from build123d import *

# Parameters (mm, degrees)
F0_W     = 100
F0_H     = 50
F1_DEPTH = 5
F2_W     = 5
F2_H     = 5
F3_DEPTH = 5
F4_W     = 5
F4_H     = 5
F5_DEPTH = 5
F6_W     = 5
F6_H     = 5
F7_DEPTH = 5


with BuildPart() as f1:
    # F0 (on Top) → F1 (new body)
    with BuildSketch(Plane.XY):
        Rectangle(F0_W, F0_H)
    extrude(amount=F1_DEPTH)

    # F2 (on face) → F3 (join)
    with BuildSketch(Plane(origin=(0, 25, 0), x_dir=(-1, 0, 0), z_dir=(0, 1, 0))):
        with Locations((0, -2.5)):
            Rectangle(F2_W, F2_H)
    extrude(amount=-F3_DEPTH)

    # F4 (on face) → F5 (join)
    with BuildSketch(Plane.XZ.offset(25)):
        with Locations((0, -2.5)):
            Rectangle(F4_W, F4_H)
    extrude(amount=-F5_DEPTH)

    # F6 (on face) → F7 (cut, through all)
    with BuildSketch(Plane.XY.offset(5)):
        Polygon((-50, 2.5), (-50, 0), (-50, -2.5), (-45, -2.5), (-45, 2.5), align=None)
        with Locations((-32.5, 0)):
            Rectangle(F6_W, F6_H)
        with Locations((32.5, 0)):
            Rectangle(F6_W, F6_H)
        Polygon((45, 2.5), (45, -2.5), (50, -2.5), (50, 0), (50, 2.5), align=None)
    extrude(amount=-F7_DEPTH, mode=Mode.SUBTRACT)


solid = f1.part
Read the model definition and answer for the solid it produces. Units are mm, in the model's axes. A direction names the side the tool comes from. Coordinates: 2 decimals unless noted, no trailing zeros. Order: outer loops, then holes, each group sorted by start corner. A loop starts at its lowest first (then second) coordinate and runs counter-clockwise, first axis right, second up. Notation, with made-up numbers: (28.25, 36.25) -> (55.25, 36.25) arc R20 cw to (55.25, 64.25) -> close; hole circle Ø1 at (-25, 50). An arc over 180 degrees is marked (long way). Answer as a JSON object with one key per item and string values.
1) Consider line 1 along Y through (x, z) = (-34.5, 4.75); line 2 along Z through (x, y) = (25.5, 12.5); line 3 along X through (y, z) = (21.5, -3.5). Determine where each line is inside the solid, lowest interval first. Write a range as from..to.
Model answer:
{"line 1": "y = -25..-2.5, 2.5..25", "line 2": "z = 0..5", "line 3": "x = -2.5..2.5"}
2) A tool of negligible diameter and unlimited length cuts with its end or side. For faces 1 (the face through (2.5, -23, -3)), 2 (the face through (48, 2.5, 3)), 3 (the face through (-2.5, 23, -3)), 4 (the face through (0, -20, -2)), from which of +Z, -Z, +X, -X, +Y, -Y can it reach the whole face along a straight path? Write none if from no direction.
Model answer:
{"face 1": "-Z, +X, +Y, -Y", "face 2": "+Z, -Z, +X", "face 3": "-Z, -X, +Y, -Y", "face 4": "-Z, +X, -X"}
3) A cutting plane is placed at C-C, the plane z = -3.75. Determine the outline of the cut face in (x, y), plus the area to 3 significant figures.
Model answer:
{"outline": "(-2.5, -25) -> (2.5, -25) -> (2.5, -20) -> (-2.5, -20) -> close; (-2.5, 20) -> (2.5, 20) -> (2.5, 25) -> (-2.5, 25) -> close", "area": "50.0 mm²"}
4) A cutting plane is placed at D-D, the plane x = -1. Determine the outline of the cut face in (y, z), plus the area to 3 significant figures.
Model answer:
{"outline": "(-25, -5) -> (-20, -5) -> (-20, 0) -> (20, 0) -> (20, -5) -> (25, -5) -> (25, 5) -> (-25, 5) -> close", "area": "300 mm²"}
5) A cutting plane is placed at B-B, the plane z = 1. Determine the outline of the cut face in (x, y), plus the area to 3 significant figures.
Model answer:
{"outline": "(-50, -25) -> (50, -25) -> (50, -2.5) -> (45, -2.5) -> (45, 2.5) -> (50, 2.5) -> (50, 25) -> (-50, 25) -> (-50, 2.5) -> (-45, 2.5) -> (-45, -2.5) -> (-50, -2.5) -> close; hole (-35, -2.5) -> (-30, -2.5) -> (-30, 2.5) -> (-35, 2.5) -> close; hole (30, -2.5) -> (35, -2.5) -> (35, 2.5) -> (30, 2.5) -> close", "area": "4,900 mm²"}
6) Each of these flat-tipped pins is pushed along its axis until it touches: pin 1 (25 mm diameter, centred on x = 5.5, y = 3.5, fed in from -Z); pin 2 (2.5 mm diameter, centred on y = -23.5, z = -1.5, fed in from +X); pin 3 (5.5 mm diameter, centred on y = -0.5, z = 2, fed in from -X); pin 4 (1.5 mm diameter, centred on y = -0.5, z = 3, fed in from +X). Where does it stop, or does it pass through?
Model answer:
{"pin 1": "stops at z = 0", "pin 2": "stops at x = 2.5", "pin 3": "stops at x = -50", "pin 4": "stops at x = 45"}
7) A cutting plane is placed at A-A, the plane y = 0.5. Determine the outline of the cut face in (x, z), plus the area to 3 significant figures.
Model answer:
{"outline": "(-45, 0) -> (-35, 0) -> (-35, 5) -> (-45, 5) -> close; (-30, 0) -> (30, 0) -> (30, 5) -> (-30, 5) -> close; (35, 0) -> (45, 0) -> (45, 5) -> (35, 5) -> close", "area": "400 mm²"}
8) The mould has two halves that part along X. Classify faces 5 (the face through (-47, 2.5, 3)), 6 (the face through (45, 0, 3)), 7 (the face through (-35, 0, 3)): released by +X, released by -X, zero draft, split by the parting line, or undercut.
Model answer:
{"face 5": "zero draft", "face 6": "released by +X", "face 7": "undercut"}
